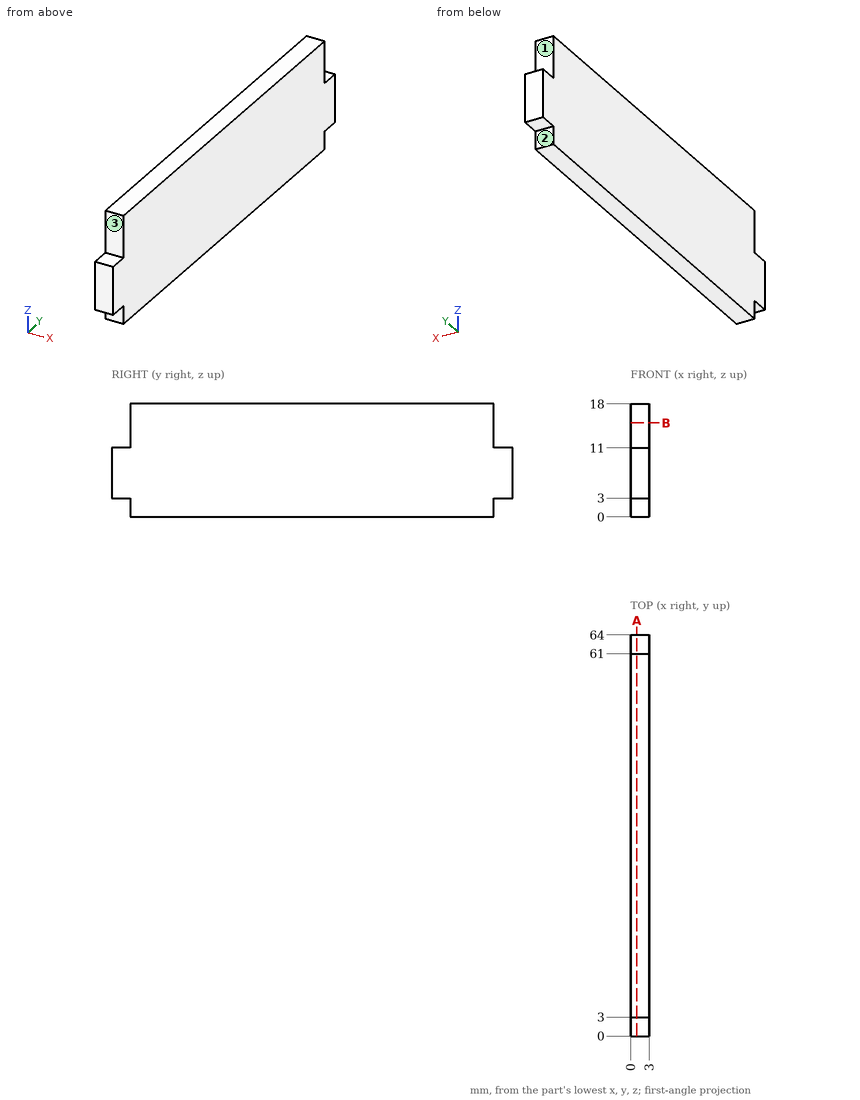
Input: dimensioned drawing with shaded views. Units: mm. Origin: part minimum x, y, z. A direction names the side the tool comes from. Give positions to 0.01 mm unless a question says otherwise; leave off trailing zeros. Loops run counter-clockwise (first coordinate to the right, second up) from the corner with the lowest first, then second, coordinate; pieces in that order, holes last. Notation, with made-up numbers: (53, 11) -> (66, 11) arc R14 cw to (66, 29) -> close; hole circle Ø5 at (6, 12.5). An arc over 180 degrees is marked (long way). Return JSON: item names as keys, results as strings.
Item 1: Pin query (flat end, axial travel): P1, Ø1.5, axis at x = 2, y = 1.5, coming from the -Z side; P2, Ø1.5, axis at x = 2, y = 2, coming from the +Z side. Return the tip coordinate at first contact, or that it passes through.
Filled in:
{"P1": "z = 3", "P2": "z = 11"}
Item 2: Section A-A, the plane x = 1. Output: boundary loops of the cut face in (y, z).
Filled in:
{"outline": "(0, 3) -> (3, 3) -> (3, 0) -> (61, 0) -> (61, 3) -> (64, 3) -> (64, 11) -> (61, 11) -> (61, 18) -> (3, 18) -> (3, 11) -> (0, 11) -> close"}
Item 3: Line query: line 1 (Y direction, x = 1.45, z = 11.75). Output: solid intervals per line, ascending.
Filled in:
{"line 1": "3 to 61"}
Item 4: Access query for the marked faces 1, 2 and 3. Directions: +Z, -Z, +X, -X, +Y, -Y. A direction counts if a zero-diameter tool reaches every point of the face in a straight line with its end or side. Return the directions, or none.
Filled in:
{"face 1": "+Z, +X, -X, +Y", "face 2": "-Z, +X, -X, +Y", "face 3": "+Z, +X, -X, -Y"}
Item 5: Section B-B, the plane z = 15. Output: boundary loops of the cut face in (x, y), plus the area to 3 significant figures.
Filled in:
{"outline": "(0, 3) -> (3, 3) -> (3, 61) -> (0, 61) -> close", "area": "174 mm^2"}
